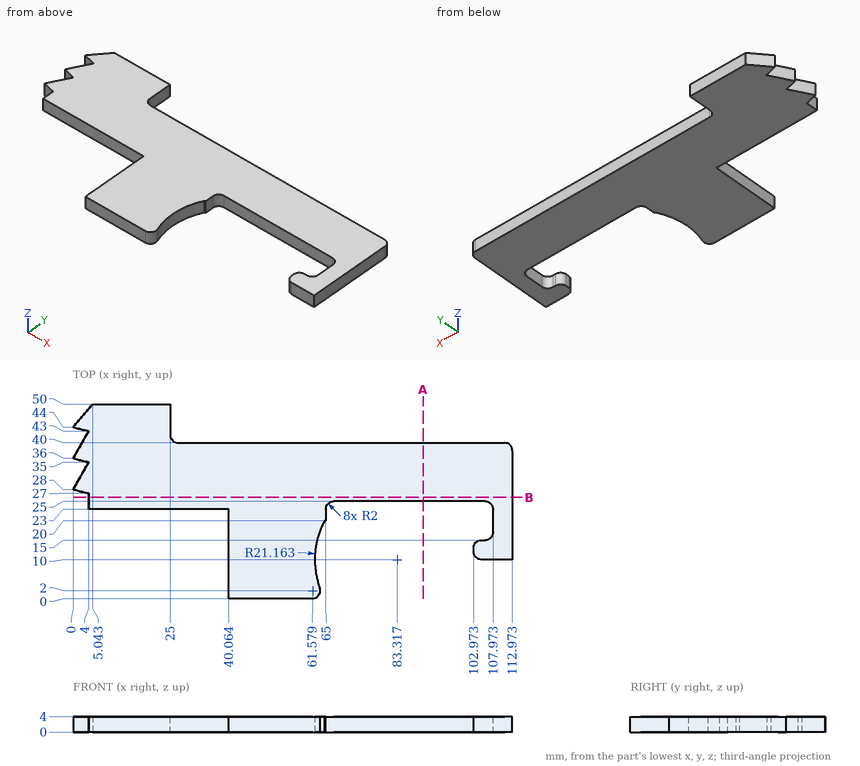
For this review, use the dimensioned drawing (mm, ordinates from the lowest corner) and the shaded views. Give positions to 0.01 mm unless a question says otherwise; leave off trailing zeros. Order: outer loops, then holes, each group sorted by start corner. A loop starts at its lowest first (then second) coordinate and runs counter-clockwise, first axis right, second up. Notation, with made-up numbers: (41, -11.5) - (84, -11.5) arc R9 cw to (84, -1.5) - close; hole circle Ø5 at (7.25, 17.25). An arc over 180 degrees is marked (long way). Use CSV: the item, a comma, the result in double quotes. Start each with the question number.
Q1. Take a section at A-A (x = 90). State the section outline as (y, z) points.
Q2. For line 1 (Y direction, x = 11, z = 1.7); line 2 (X direction, y = 23.5, z = 0.45); line 3 (Y direction, x = 93, z = 3.1), list the stretches that pass through material, from the lowest coordinate up.
Q3. Take a section at B-B (y = 26). State the section outline as (x, z) points.
Q4. For P1, Ø2, axis at y = 45.5, z = 2, coming from the +X side; P2, Ø1.2, axis at y = 19.5, z = 2.5, coming from the -X side; P3, Ø1.2, axis at x = 67, z = 1.5, coming from the +Y side, all flat-tipped, find the tip position at first contact; note any pin that passes through.
Calculated:
1,outline,"(25, 0) - (40, 0) - (40, 4) - (25, 4) - close"
2,line 1,"y = 23 to 50"
2,line 2,"x = 4 to 65.06, 107.91 to 112.97"
2,line 3,"y = 25 to 40"
3,outline,"(4, 0) - (112.97, 0) - (112.97, 4) - (4, 4) - close"
4,P1,"stops at x = 25"
4,P2,"stops at x = 40.06"
4,P3,"stops at y = 40"
